from build123d import *

# Parameters (mm, degrees)
SKETCH_1_R      = 15
EXTRUDE_1_DEPTH = 2


with BuildPart() as part:
    # 草图1 → 凸台-拉伸1 (new body)
    with BuildSketch(Plane(origin=(0, 0, 0), x_dir=(1, 0, 0), z_dir=(0, 1, 0))):
        Polygon((0, -1), (30, -1), (30, 1), (70, 1), (70, -1), (100, -1), (100, 30), (102, 30), (102, 70), (100, 70), (100, 100), (0, 100), (0, 70), (-2, 70), (-2, 30), (0, 30), align=None)
        with Locations(Location((50, 50, 0), (0, 0, 270))):
            Circle(SKETCH_1_R, mode=Mode.SUBTRACT)
    extrude(amount=EXTRUDE_1_DEPTH)


solid = part.part
Verification items for the finished model (mm, model axes). Round coordinates to 2 decimals unless told otherwise and drop trailing zeros. Write each loop counter-clockwise with the first axis right and the second up, starting at its lowest first coordinate (ties: lowest second). Pieces come first, ordered by that corner, then holes.
(1) Section check A-A (z = -50). Enter the section's corners in (x, y), plus the area to 3 significant figures.
Returned:
outline: (-2, 0) - (35, 0) - (35, 2) - (-2, 2) - close; (65, 0) - (102, 0) - (102, 2) - (65, 2) - close
area: 148 mm2
(2) Mould release check, pull along X, two halves, no side actions. Record for faces 1 (the flat face through (61, 0, -61)), 2 (the cylindrical face through (60.138, 0.986, -61.056)): pulls with the +X half, pulls with the -X half, needs draft (parallel to the pull), parting line crosses it, or undercut.
Returned:
face 1: needs draft
face 2: undercut
(3) Section check D-D (z = -84.5). Enter the section's corners in (x, y), plus the area to 3 significant figures.
Returned:
outline: (0, 0) - (100, 0) - (100, 2) - (0, 2) - close
area: 200 mm2
(4) Section check B-B (x = 50). Enter the section's corners in (y, z).
Returned:
outline: (0, -100) - (2, -100) - (2, -65) - (0, -65) - close; (0, -35) - (2, -35) - (2, -1) - (0, -1) - close
(5) Section check C-C (y = 1.5). Enter the section's corners in (x, z), plus the area to 3 significant figures.
Returned:
outline: (-2, -70) - (0, -70) - (0, -100) - (100, -100) - (100, -70) - (102, -70) - (102, -30) - (100, -30) - (100, 1) - (70, 1) - (70, -1) - (30, -1) - (30, 1) - (0, 1) - (0, -30) - (-2, -30) - close; hole circle Ø30 at (50, -50)
area: 9,470 mm2
(6) Material ranges on line 1 (X direction, y = 0.65, z = -50); line 2 (X direction, y = 1.1, z = -4.5); line 3 (Z direction, x = 51, y = 1.2), recorded low to high.
Returned:
line 1: x = -2 to 35, 65 to 102
line 2: x = 0 to 100
line 3: z = -100 to -64.97, -35.03 to -1
(7) Depth check by flat-ended pin: pin 1 Ø0.6 at (x, y) = (-1, 1) entering from +Z; pin 2 Ø1 at (y, z) = (0.5, 0) entering from -X; pin 3 Ø0.6 at (y, z) = (1, -18) entering from +X. Enter the tip coordinate at first touch or a pass-through.
Returned:
pin 1: stops at z = -30
pin 2: stops at x = 0
pin 3: stops at x = 100
